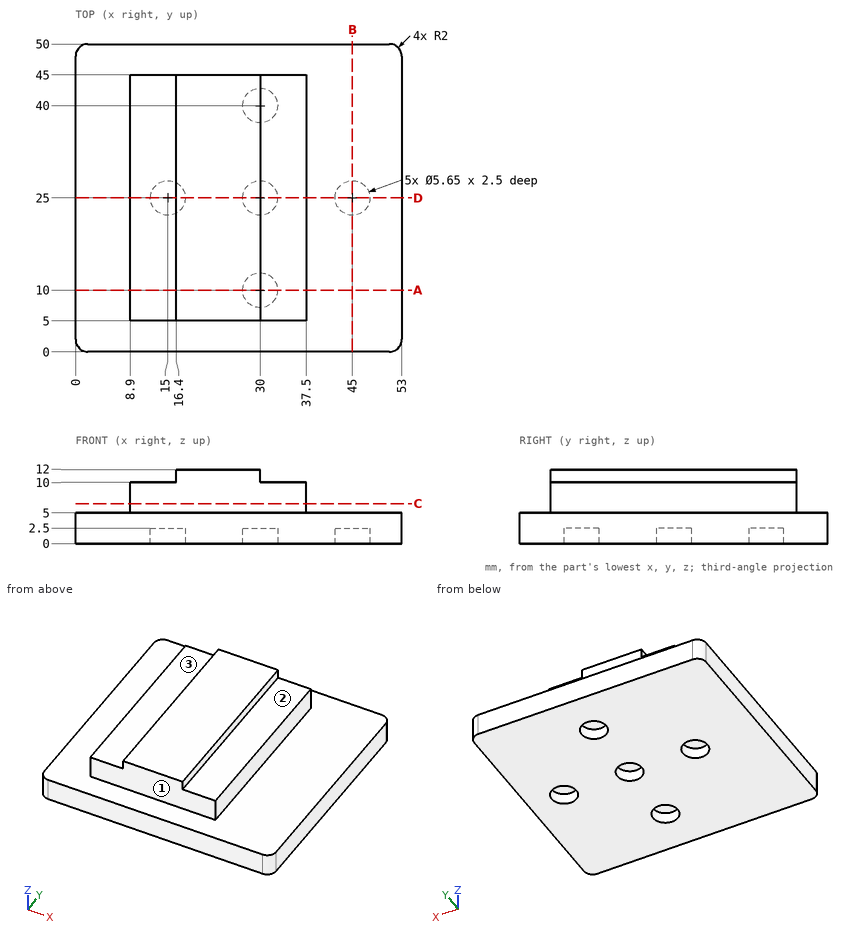
Check sheet for the drawn part. Datum: minimum x, y, z corner. Units: mm. A direction names the side the tool comes from. Round coordinates to 2 decimals unless told otherwise and drop trailing zeros. Loops run counter-clockwise (first coordinate to the right, second up) from the corner with the lowest first, then second, coordinate; pieces in that order, holes last.
Item 1: Cross-section at B-B on x = 45. Record the boundary of the cut face in (y, z) (3 decimals), then the cut area to 3 significant figures.
Item 2: Cross-section at A-A on y = 10. Record the boundary of the cut face in (x, z) (3 decimals).
Item 3: Cross-section at C-C on z = 6.5. Record the boundary of the cut face in (x, y).
Item 4: Thickness scan on line 1 (Y direction, x = 30, z = 0.7) (3 decimals); line 2 (Y direction, x = 15, z = 1.5) (3 decimals); line 3 (Z direction, x = 31, y = 40). Record the ranges inside material, lowest first.
Item 5: Cross-section at D-D on y = 25. Record the boundary of the cut face in (x, z) (3 decimals), then the cut area to 3 significant figures.
Item 6: Access from +Z, -Z, +X, -X, +Y, -Y to the whole of each face (thin tool, end or side, straight path). Record for the marked faces 1, 2 and 3.
Item 7: Gauge pin test, flat ends, axial feed: pin 1 (1.5 mm diameter, centred on y = 15.5, z = 6.5, fed in from +X); pin 2 (3 mm diameter, centred on x = 31, y = 24.5, fed in from -Z); pin 3 (5 mm diameter, centred on x = 30.5, z = 10.5, fed in from -Y). Record the tip position at first contact, or that the pin passes through.
Answer sheet:
1. outline: (0, 0) - (22.175, 0) - (22.175, 2.5) - (27.825, 2.5) - (27.825, 0) - (50, 0) - (50, 5) - (0, 5) - close
1. area: 236 mm2
2. outline: (0, 0) - (27.175, 0) - (27.175, 2.5) - (32.825, 2.5) - (32.825, 0) - (53, 0) - (53, 5) - (37.5, 5) - (37.5, 10) - (30, 10) - (30, 12) - (16.4, 12) - (16.4, 10) - (8.9, 10) - (8.9, 5) - (0, 5) - close
3. outline: (8.9, 5) - (37.5, 5) - (37.5, 45) - (8.9, 45) - close
4. line 1: y = 0 to 7.175, 12.825 to 22.175, 27.825 to 37.175, 42.825 to 50
4. line 2: y = 0 to 22.175, 27.825 to 50
4. line 3: z = 2.5 to 10
5. outline: (0, 0) - (12.175, 0) - (12.175, 2.5) - (17.825, 2.5) - (17.825, 0) - (27.175, 0) - (27.175, 2.5) - (32.825, 2.5) - (32.825, 0) - (42.175, 0) - (42.175, 2.5) - (47.825, 2.5) - (47.825, 0) - (53, 0) - (53, 5) - (37.5, 5) - (37.5, 10) - (30, 10) - (30, 12) - (16.4, 12) - (16.4, 10) - (8.9, 10) - (8.9, 5) - (0, 5) - close
5. area: 393 mm2
6. face 1: +Z, +X, -X, -Y
6. face 2: +Z, +X, +Y, -Y
6. face 3: +Z, -X, +Y, -Y
7. pin 1: stops at x = 37.5
7. pin 2: stops at z = 2.5
7. pin 3: stops at y = 5
